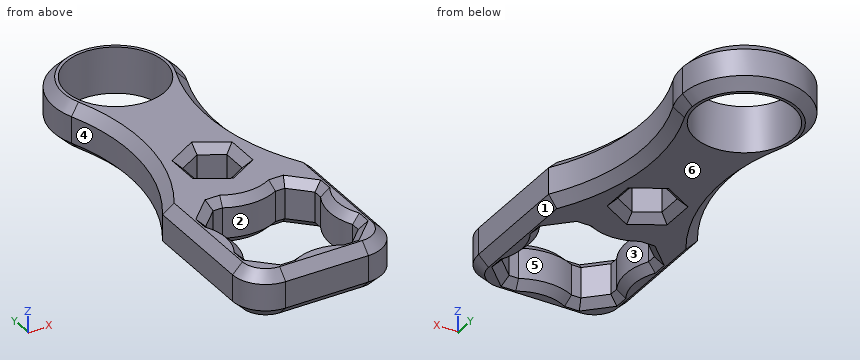
```python
from build123d import *

# Parameters (mm, degrees)
F0_W     = 22.5
F0_H     = 22.5
F0_R     = 7.4115696456
F1_DEPTH = 7
F2_SIZE  = 1.2
F3_R     = 5
F4_SIZE  = 1.5
F5_SCALE = 1.05


with BuildPart() as f1:
    # F0 (on Top) → F1 (new body)
    with BuildSketch(Plane.XY):
        Rectangle(F0_W, F0_H)
        with BuildLine():
            Line((4, 8.25), (5.4215728753, 8.25))
            Line((5.4215728753, 8.25), (8.25, 5.4215728753))
            Line((8.25, 5.4215728753), (8.25, 4))
            ThreePointArc((8.25, 4), (7.25, 0), (8.25, -4))
            Line((8.25, -4), (8.25, -5.4215728753))
            Line((8.25, -5.4215728753), (5.4215728753, -8.25))
            Line((5.4215728753, -8.25), (4, -8.25))
            ThreePointArc((4, -8.25), (0, -7.25), (-4, -8.25))
            Line((-4, -8.25), (-5.4215728753, -8.25))
            Line((-5.4215728753, -8.25), (-8.25, -5.4215728753))
            Line((-8.25, -5.4215728753), (-8.25, -4))
            ThreePointArc((-8.25, -4), (-7.25, 0), (-8.25, 4))
            Line((-8.25, 4), (-8.25, 5.4215728753))
            Line((-8.25, 5.4215728753), (-5.4215728753, 8.25))
            Line((-5.4215728753, 8.25), (-4, 8.25))
            ThreePointArc((-4, 8.25), (0, 7.25), (4, 8.25))
        make_face(mode=Mode.SUBTRACT)
        with BuildLine():
            Line((-11.25, 11.25), (11.25, 11.25))
            ThreePointArc((11.25, 11.25), (6.7870639403, 24.4144327009), (8.7322033942, 38.1780266762))
            ThreePointArc((8.7322033942, 38.1780266762), (0, 32.2246467329), (-8.7322033942, 38.1780266762))
            ThreePointArc((-8.7322033942, 38.1780266762), (-6.7870639403, 24.4144327009), (-11.25, 11.25))
        make_face()
        Polygon((3.33375, 15.4506308903), (0, 13.5258894304), (-3.33375, 15.4506308903), (-3.33375, 19.3001138101), (0, 21.22485527), (3.33375, 19.3001138101), align=None, mode=Mode.SUBTRACT)
        with BuildLine():
            ThreePointArc((-8.7322033942, 38.1780266762), (0, 32.2246467329), (8.7322033942, 38.1780266762))
            ThreePointArc((8.7322033942, 38.1780266762), (9.2171730729, 39.8612931132), (9.3807307723, 41.6053775052))
            ThreePointArc((9.3807307723, 41.6053775052), (-1.744084392, 50.8225505781), (-8.7322033942, 38.1780266762))
        make_face()
        with Locations((0, 41.6053775052)):
            Circle(F0_R, mode=Mode.SUBTRACT)
    extrude(amount=F1_DEPTH)

    # F2
    f2_edges = [f1.edges().sort_by_distance(p)[0] for p in [
        (-7.25, 0, 7),
        (-8.25, 4.710786, 7),
        (-6.835786, 6.835786, 7),
        (-4.710786, 8.25, 7),
        (0, 7.25, 7),
        (4.710786, 8.25, 7),
        (6.835786, 6.835786, 7),
        (8.25, 4.710786, 7),
        (7.25, 0, 7),
        (8.25, -4.710786, 7),
        (6.835786, -6.835786, 7),
        (4.710786, -8.25, 7),
        (0, -7.25, 7),
        (-4.710786, -8.25, 7),
        (-6.835786, -6.835786, 7),
        (-8.25, -4.710786, 7),
        (1.666875, 14.48826, 7),
        (-1.666875, 14.48826, 7),
        (-3.33375, 17.375372, 7),
        (-1.666875, 20.262485, 7),
        (1.666875, 20.262485, 7),
        (3.33375, 17.375372, 7),
        (-1.666875, 14.48826, 0),
        (1.666875, 14.48826, 0),
        (3.33375, 17.375372, 0),
        (1.666875, 20.262485, 0),
        (-1.666875, 20.262485, 0),
        (0, -7.25, 0),
        (-4.710786, -8.25, 0),
        (-6.835786, -6.835786, 0),
        (-8.25, -4.710786, 0),
        (-7.25, 0, 0),
        (-8.25, 4.710786, 0),
        (-4.710786, 8.25, 0),
        (4.710786, 8.25, 0),
        (-6.835786, 6.835786, 0),
        (0, 7.25, 0),
        (6.835786, 6.835786, 0),
        (8.25, 4.710786, 0),
        (7.25, 0, 0),
        (8.25, -4.710786, 0),
        (6.835786, -6.835786, 0),
        (4.710786, -8.25, 0),
        (-3.33375, 17.375372, 0),
    ]]
    chamfer(f2_edges, length=F2_SIZE)

    # F3
    f3_edges = [f1.edges().sort_by_distance(p)[0] for p in [
        (11.25, -11.25, 3.5),
        (-11.25, -11.25, 3.5),
    ]]
    fillet(f3_edges, radius=F3_R)

    # F4
    f4_edges = [f1.edges().sort_by_distance(p)[0] for p in [
        (0, 50.986108, 7),
        (11.25, 2.5, 7),
        (0, -11.25, 7),
        (-11.25, 2.5, 7),
        (0, 50.986108, 0),
        (-11.25, 2.5, 0),
        (0, -11.25, 0),
        (11.25, 2.5, 0),
    ]]
    chamfer(f4_edges, length=F4_SIZE)


with BuildPart() as f1_1:
    # F5: moved
    add(f1.part.scale(F5_SCALE))


solid = f1_1.part
```
Can you work these out from the model? Positions are in its coordinate system, mm. Face numbers are marked on the shaded views. A direction names the side the tool comes from. Round coordinates to 2 decimals unless told otherwise and drop trailing zeros.
Item 1: Please list where these lines run through material, in increasing order: L1, parallel to Y at x = 0, z = 2; L2, parallel to Y at x = -1.25, z = 4; L3, parallel to Y at x = -6, z = 5.5.
Item 2: Which directions (+Z, -Z, +X, -X, +Y, -Y) give clear straight access to the entire face, cutting with the end or side of a thin tool? Please do the marked faces 1 and 2.
Item 3: Suppose I cut it at B-B, the plane z = 2.75. State how many separate pieces and enclosed holes the cut face has, then the cut area to 3 significant figures.
Item 4: Will these pins go through, and if not, where does the flat tip stop? pin 1 Ø9.5 at (x, y) = (0, 43.69) entering from -Z; pin 2 Ø1.5 at (y, z) = (36.5, 5) entering from -X; pin 3 Ø2 at (y, z) = (41, 4.5) entering from +X; pin 4 Ø1.2 at (x, z) = (-5, 3.5) entering from +Y.
Item 5: If we mould it in two halves opening along X, with no side actions, what happens to the marked faces 3, 4, 5 and 6? For each: +X half, -X half, draft (parallel to the pull), parting line (faces both ways), or undercut.
Reported:
1. L1: y = -11.81 to -7.61, 7.61 to 14.2, 22.29 to 35.9, 51.47 to 53.54
1. L2: y = -11.81 to -7.7, 7.7 to 14.92, 21.56 to 36, 51.37 to 53.46
1. L3: y = -11.81 to -8.36, 8.36 to 38.73, 48.64 to 51.5
2. face 1: -Z, +X, +Y, -Y
2. face 2: +Z, -Z
3. separate pieces: 1
3. enclosed holes: 3
3. area: 740 mm2
4. pin 1: passes through
4. pin 2: stops at x = -8.21
4. pin 3: stops at x = 9.7
4. pin 4: stops at y = 52.5
5. face 3: undercut
5. face 4: -X half
5. face 5: undercut
5. face 6: draft
